Verification items for the finished model (mm, model axes). Face numbers are marked on the shaded views. A direction names the side the tool comes from. Round coordinates to 2 decimals unless told otherwise and drop trailing zeros. Loops run counter-clockwise (first coordinate to the right, second up) from the corner with the lowest first, then second, coordinate; pieces in that order, holes last. Notation, with made-up numbers: (-24.75, 33.25) -> (-0.75, 33.25) arc R32 cw to (-0.75, 71.25) -> close; hole circle Ø6 at (23.5, -11). An arc over 180 degrees is marked (long way). Write item = value, one per line. Start each with the question number.
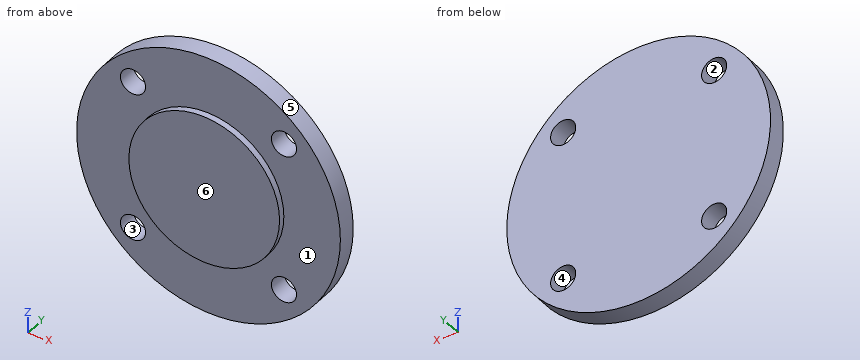
```python
from build123d import *

# Parameters (mm, degrees)
SKETCH1_R                = 21
SKETCH1_R_2              = 12
SKETCH1_R_3              = 2
BOSS_EXTRUDE1_DEPTH      = 3
SKETCH1_2_R              = 12
BOSS_EXTRUDE2_DEPTH      = 3
BOSS_EXTRUDE2_DEPTH_BACK = 1


with BuildPart() as part:
    # Sketch1 → Boss-Extrude1 (new body)
    with BuildSketch(Plane(origin=(0, 0, 0), x_dir=(1, 0, 0), z_dir=(0, 1, 0))):
        Circle(SKETCH1_R)
        Circle(SKETCH1_R_2, mode=Mode.SUBTRACT)
        with Locations((-12.02081528, 12.02081528)):
            Circle(SKETCH1_R_3, mode=Mode.SUBTRACT)
        with Locations((12.02081528, 12.02081528)):
            Circle(SKETCH1_R_3, mode=Mode.SUBTRACT)
        with Locations((12.02081528, -12.02081528)):
            Circle(SKETCH1_R_3, mode=Mode.SUBTRACT)
        with Locations((-12.02081528, -12.02081528)):
            Circle(SKETCH1_R_3, mode=Mode.SUBTRACT)
    extrude(amount=BOSS_EXTRUDE1_DEPTH)

    # Sketch1_2 → Boss-Extrude2 (add, two sides)
    with BuildSketch(Plane(origin=(0, 0, 0), x_dir=(1, 0, 0), z_dir=(0, 1, 0))) as boss_extrude2_sk:
        Circle(SKETCH1_2_R)
    extrude(amount=BOSS_EXTRUDE2_DEPTH)
    extrude(boss_extrude2_sk.sketch, amount=-BOSS_EXTRUDE2_DEPTH_BACK)


solid = part.part
```
(1) Section check B-B on x = 0. Enter the section's corners in (y, z).
(2) Section check D-D on y = 1.6. Enter the section's corners in (x, z), then the cut area to 3 significant figures.
(3) Scan lines: line 1 (X direction, y = 0.35, z = 13); line 2 (Y direction, x = 8, z = -9.5). Record each from-to range of solid material in increasing order. Write a range as [from, to].
(4) Depth check by flat-ended pin: pin 1 Ø1.5 at (x, y) = (-5.5, 0) entering from -Z; pin 2 Ø2 at (x, y) = (14.5, 0) entering from -Z; pin 3 Ø12 at (x, z) = (16.5, 13) entering from -Y. Enter the tip coordinate at first touch or a pass-through.
(5) Access from +Z, -Z, +X, -X, +Y, -Y to the whole of each face (thin tool, end or side, straight path). Record for the marked faces 1 and 2.
(6) Section check C-C on x = 11.5. Enter the section's corners in (y, z).
(7) Section check A-A on z = 0. Enter the section's corners in (x, y), then the cut area to 3 significant figures.
(8) Draft check along X on the marked faces 3, 4, 5 and 6. Enter one of: +X half, -X half, draft (parallel to the pull), parting line (faces both ways), or undercut.
Computed values:
q1.outline = (-1, -12) -> (0, -12) -> (0, -21) -> (3, -21) -> (3, 21) -> (0, 21) -> (0, 12) -> (-1, 12) -> close
q2.outline = circle Ø42 at (0, 0); hole circle Ø4 at (-12.02, -12.02); hole circle Ø4 at (-12.02, 12.02); hole circle Ø4 at (12.02, -12.02); hole circle Ø4 at (12.02, 12.02)
q2.area = 1,340 mm²
q3.line_1 = [-16.49, -13.76], [-10.28, 10.28], [13.76, 16.49]
q3.line_2 = [0, 3]
q4.pin_1 = -20.46
q4.pin_2 = -16.09
q4.pin_3 = 0
q5.face_1 = -Y
q5.face_2 = +Y, -Y
q6.outline = (-1, -3.43) -> (0, -3.43) -> (0, -10.09) -> (3, -10.09) -> (3, 10.09) -> (0, 10.09) -> (0, 3.43) -> (-1, 3.43) -> close; (0, -17.57) -> (3, -17.57) -> (3, -13.95) -> (0, -13.95) -> close; (0, 13.95) -> (3, 13.95) -> (3, 17.57) -> (0, 17.57) -> close
q7.outline = (-21, 0) -> (-12, 0) -> (-12, -1) -> (12, -1) -> (12, 0) -> (21, 0) -> (21, 3) -> (-21, 3) -> close
q7.area = 150 mm²
q8.face_3 = undercut
q8.face_4 = undercut
q8.face_5 = parting line
q8.face_6 = draft
